```python
from build123d import *

# Parameters (mm, degrees)
SKETCH2_R           = 25
BOSS_EXTRUDE1_DEPTH = 12


with BuildPart() as part:
    # Sketch2 → Boss-Extrude1 (new body)
    with BuildSketch(Plane.XY):
        with BuildLine():
            Line((-2.137931034, 28.911787374), (1.862068966, 28.911787374))
            Line((1.862068966, 28.911787374), (1.862068966, 26.935714194))
            ThreePointArc((1.862068966, 26.935714194), (2.42026134, 26.891305938), (2.977412735, 26.835331438))
            Line((2.977412735, 26.835331438), (3.058825373, 28.828905384))
            Line((3.058825373, 28.828905384), (6.994543728, 28.114677805))
            Line((6.994543728, 28.114677805), (6.641702237, 26.170360934))
            ThreePointArc((6.641702237, 26.170360934), (7.18299483, 26.026997239), (7.72119794, 25.87243905))
            Line((7.72119794, 25.87243905), (8.157268617, 27.819438654))
            Line((8.157268617, 27.819438654), (11.9022081, 26.413939357))
            Line((11.9022081, 26.413939357), (11.207865734, 24.563870739))
            ThreePointArc((11.207865734, 24.563870739), (11.714860956, 24.326159433), (12.21681749, 24.077985182))
            Line((12.21681749, 24.077985182), (12.993530536, 25.915832275))
            Line((12.993530536, 25.915832275), (16.42732571, 23.864235166))
            Line((16.42732571, 23.864235166), (15.413799204, 22.167877528))
            ThreePointArc((15.413799204, 22.167877528), (15.870201812, 21.843458848), (16.319778474, 21.509645059))
            Line((16.319778474, 21.509645059), (17.412169691, 23.179269724))
            Line((17.412169691, 23.179269724), (20.424455555, 20.54751482))
            Line((20.424455555, 20.54751482), (19.124320485, 19.059390494))
            ThreePointArc((19.124320485, 19.059390494), (19.515461323, 18.658691523), (19.89820835, 18.249967246))
            Line((19.89820835, 18.249967246), (21.271167387, 19.697706372))
            Line((21.271167387, 19.697706372), (23.765126594, 16.570380442))
            Line((23.765126594, 16.570380442), (22.22017037, 15.338318966))
            ThreePointArc((22.22017037, 15.338318966), (22.53347785, 14.874218499), (22.837093437, 14.403720469))
            Line((22.837093437, 14.403720469), (24.44649226, 15.583042529))
            Line((24.44649226, 15.583042529), (26.34196691, 12.060660402))
            Line((26.34196691, 12.060660402), (24.601845697, 11.124261247))
            ThreePointArc((24.601845697, 11.124261247), (24.827249859, 10.611675855), (25.041975551, 10.094526265))
            Line((25.041975551, 10.094526265), (26.836086758, 10.967526878))
            Line((26.836086758, 10.967526878), (28.072154735, 7.163300813))
            Line((28.072154735, 7.163300813), (26.192797461, 6.552660618))
            ThreePointArc((26.192797461, 6.552660618), (26.323053629, 6.008065217), (26.441987966, 5.460885681))
            Line((26.441987966, 5.460885681), (28.363147346, 5.999505889))
            Line((28.363147346, 5.999505889), (28.900080409, 2.035706842))
            Line((28.900080409, 2.035706842), (26.941891163, 1.770452086))
            ThreePointArc((26.941891163, 1.770452086), (26.972812797, 1.211350419), (26.992133131, 0.651727738))
            Line((26.992133131, 0.651727738), (28.978593042, 0.838655845))
            Line((28.978593042, 0.838655845), (28.79913372, -3.157316422))
            Line((28.79913372, -3.157316422), (26.825050314, -3.068660234))
            ThreePointArc((26.825050314, -3.068660234), (26.755643568, -3.624298177), (26.674728928, -4.17837727))
            Line((26.674728928, -4.17837727), (28.662642913, -4.349149289))
            Line((28.662642913, -4.349149289), (27.772559177, -8.248860938))
            Line((27.772559177, -8.248860938), (25.846030277, -7.809143288))
            ThreePointArc((25.846030277, -7.809143288), (25.67852594, -8.343458848), (25.499976989, -8.874185796))
            Line((25.499976989, -8.874185796), (27.425451857, -9.397169186))
            Line((27.425451857, -9.397169186), (25.853351731, -13.075280276))
            Line((25.853351731, -13.075280276), (24.036297561, -12.298634052))
            ThreePointArc((24.036297561, -12.298634052), (23.77607936, -12.794453887), (23.505634809, -13.284770688))
            Line((23.505634809, -13.284770688), (25.306784213, -14.143156333))
            Line((25.306784213, -14.143156333), (23.103196288, -17.481449348))
            Line((23.103196288, -17.481449348), (21.454018464, -16.392836598))
            ThreePointArc((21.454018464, -16.392836598), (21.109450027, -16.83422465), (20.755802185, -17.268372119))
            Line((20.755802185, -17.268372119), (22.374735702, -18.434570799))
            Line((22.374735702, -18.434570799), (19.610485106, -21.325750254))
            Line((19.610485106, -21.325750254), (18.182189561, -19.960159888))
            ThreePointArc((18.182189561, -19.960159888), (17.7643456, -20.332929582), (17.338861001, -20.696953862))
            Line((17.338861001, -20.696953862), (18.723544776, -22.133482991))
            Line((18.723544776, -22.133482991), (15.487476798, -24.484624))
            Line((15.487476798, -24.484624), (14.325970126, -22.885947216))
            ThreePointArc((14.325970126, -22.885947216), (13.84828049, -23.178117427), (13.364634558, -23.460318479))
            Line((13.364634558, -23.460318479), (14.470563714, -25.121006829))
            Line((14.470563714, -25.121006829), (10.866688243, -26.856541785))
            Line((10.866688243, -26.856541785), (10.009302223, -25.076161369))
            ThreePointArc((10.009302223, -25.076161369), (9.48712025, -25.278341507), (8.960857764, -25.469649156))
            Line((8.960857764, -25.469649156), (9.752486829, -27.301120837))
            Line((9.752486829, -27.301120837), (5.896635386, -28.365268219))
            Line((5.896635386, -28.365268219), (5.370927111, -26.460407064))
            ThreePointArc((5.370927111, -26.460407064), (4.82103616, -26.566098892), (4.269071629, -26.660364353))
            Line((4.269071629, -26.660364353), (4.720956992, -28.603754358))
            Line((4.720956992, -28.603754358), (0.737059816, -28.962311594))
            Line((0.737059816, -28.962311594), (0.559925982, -26.994193503))
            ThreePointArc((0.559925982, -26.994193503), (0, -27), (-0.559925982, -26.994193503))
            Line((-0.559925982, -26.994193503), (-0.462308287, -28.987039679))
            Line((-0.462308287, -28.987039679), (-4.446205463, -28.628482443))
            Line((-4.446205463, -28.628482443), (-4.269071629, -26.660364353))
            ThreePointArc((-4.269071629, -26.660364353), (-4.82103616, -26.566098892), (-5.370927111, -26.460407064))
            Line((-5.370927111, -26.460407064), (-5.630714597, -28.438657694))
            Line((-5.630714597, -28.438657694), (-9.48656604, -27.374510312))
            Line((-9.48656604, -27.374510312), (-8.960857764, -25.469649156))
            ThreePointArc((-8.960857764, -25.469649156), (-9.48712025, -25.278341507), (-10.009302223, -25.076161369))
            Line((-10.009302223, -25.076161369), (-10.618145107, -26.976233851))
            Line((-10.618145107, -26.976233851), (-14.222020578, -25.240698895))
            Line((-14.222020578, -25.240698895), (-13.364634558, -23.460318479))
            ThreePointArc((-13.364634558, -23.460318479), (-13.84828049, -23.178117427), (-14.325970126, -22.885947216))
            Line((-14.325970126, -22.885947216), (-15.264299696, -24.646771656))
            Line((-15.264299696, -24.646771656), (-18.500367674, -22.295630647))
            Line((-18.500367674, -22.295630647), (-17.338861001, -20.696953862))
            ThreePointArc((-17.338861001, -20.696953862), (-17.7643456, -20.332929582), (-18.182189561, -19.960159888))
            Line((-18.182189561, -19.960159888), (-19.419847134, -21.525141941))
            Line((-19.419847134, -21.525141941), (-22.18409773, -18.633962486))
            Line((-22.18409773, -18.633962486), (-20.755802185, -17.268372119))
            ThreePointArc((-20.755802185, -17.268372119), (-21.109450027, -16.83422465), (-21.454018464, -16.392836598))
            Line((-21.454018464, -16.392836598), (-22.951224707, -17.711676453))
            Line((-22.951224707, -17.711676453), (-25.154812632, -14.373383438))
            Line((-25.154812632, -14.373383438), (-23.505634809, -13.284770688))
            ThreePointArc((-23.505634809, -13.284770688), (-23.77607936, -12.794453887), (-24.036297561, -12.298634052))
            Line((-24.036297561, -12.298634052), (-25.744931032, -13.32894311))
            Line((-25.744931032, -13.32894311), (-27.317031159, -9.65083202))
            Line((-27.317031159, -9.65083202), (-25.499976989, -8.874185796))
            ThreePointArc((-25.499976989, -8.874185796), (-25.67852594, -8.343458848), (-25.846030277, -7.809143288))
            Line((-25.846030277, -7.809143288), (-27.711174092, -8.517806569))
            Line((-27.711174092, -8.517806569), (-28.601257828, -4.61809492))
            Line((-28.601257828, -4.61809492), (-26.674728928, -4.17837727))
            ThreePointArc((-26.674728928, -4.17837727), (-26.755643568, -3.624298177), (-26.825050314, -3.068660234))
            Line((-26.825050314, -3.068660234), (-28.786757215, -3.432900716))
            Line((-28.786757215, -3.432900716), (-28.966216537, 0.56307155))
            Line((-28.966216537, 0.56307155), (-26.992133131, 0.651727738))
            ThreePointArc((-26.992133131, 0.651727738), (-26.972812797, 1.211350419), (-26.941891163, 1.770452086))
            Line((-26.941891163, 1.770452086), (-28.937110276, 1.762341391))
            Line((-28.937110276, 1.762341391), (-28.400177213, 5.726140438))
            Line((-28.400177213, 5.726140438), (-26.441987966, 5.460885681))
            ThreePointArc((-26.441987966, 5.460885681), (-26.323053629, 6.008065217), (-26.192797461, 6.552660618))
            Line((-26.192797461, 6.552660618), (-28.157400803, 6.900940395))
            Line((-28.157400803, 6.900940395), (-26.921332825, 10.70516646))
            Line((-26.921332825, 10.70516646), (-25.041975551, 10.094526265))
            ThreePointArc((-25.041975551, 10.094526265), (-24.827249859, 10.611675855), (-24.601845697, 11.124261247))
            Line((-24.601845697, 11.124261247), (-26.4726893, 11.817737496))
            Line((-26.4726893, 11.817737496), (-24.57721465, 15.340119624))
            Line((-24.57721465, 15.340119624), (-22.837093437, 14.403720469))
            ThreePointArc((-22.837093437, 14.403720469), (-22.53347785, 14.874218499), (-22.22017037, 15.338318966))
            Line((-22.22017037, 15.338318966), (-23.937123781, 16.354702791))
            Line((-23.937123781, 16.354702791), (-21.443164573, 19.482028721))
            Line((-21.443164573, 19.482028721), (-19.89820835, 18.249967246))
            ThreePointArc((-19.89820835, 18.249967246), (-19.515461323, 18.658691523), (-19.124320485, 19.059390494))
            Line((-19.124320485, 19.059390494), (-20.632199408, 20.366014482))
            Line((-20.632199408, 20.366014482), (-17.619913544, 22.997769386))
            Line((-17.619913544, 22.997769386), (-16.319778474, 21.509645059))
            ThreePointArc((-16.319778474, 21.509645059), (-15.870201812, 21.843458848), (-15.413799204, 22.167877528))
            Line((-15.413799204, 22.167877528), (-16.66413917, 23.72274571))
            Line((-16.66413917, 23.72274571), (-13.230343996, 25.774342819))
            Line((-13.230343996, 25.774342819), (-12.21681749, 24.077985182))
            ThreePointArc((-12.21681749, 24.077985182), (-11.714860956, 24.326159433), (-11.207865734, 24.563870739))
            Line((-11.207865734, 24.563870739), (-12.160479788, 26.317008371))
            Line((-12.160479788, 26.317008371), (-8.415540306, 27.722507668))
            Line((-8.415540306, 27.722507668), (-7.72119794, 25.87243905))
            ThreePointArc((-7.72119794, 25.87243905), (-7.18299483, 26.026997239), (-6.641702237, 26.170360934))
            Line((-6.641702237, 26.170360934), (-7.26597258, 28.06542073))
            Line((-7.26597258, 28.06542073), (-3.330254225, 28.779648309))
            Line((-3.330254225, 28.779648309), (-2.977412735, 26.835331438))
            ThreePointArc((-2.977412735, 26.835331438), (-2.42026134, 26.891305938), (-1.862068966, 26.935714194))
            Line((-1.862068966, 26.935714194), (-2.137931034, 28.911787374))
        make_face()
        Circle(SKETCH2_R, mode=Mode.SUBTRACT)
    extrude(amount=BOSS_EXTRUDE1_DEPTH)


solid = part.part
```
Verification items for the finished model (mm, model axes). A direction names the side the tool comes from. Coordinates: 2 decimals unless noted, no trailing zeros. Answer as a JSON object with one key per item and string values. Group by question number.
(1) Gauge pin test, flat ends, axial feed: pin 1 (8 mm diameter, centred on x = 18.5, y = -3, fed in from -Z); pin 2 (2 mm diameter, centred on y = 12, z = 4.5, fed in from +X); pin 3 (1 mm diameter, centred on y = -21, z = 7.5, fed in from +X). Record the tip position at first contact, or that the pin passes through.
(2) Tool access check on faces 1 (the face through (-27.993, 0.607, 5.916)), 2 (the face through (24.394, -13.708, 5.916)), 3 (the face through (12.69, -25.98, 5.92)), 4 (the face through (5.64, -27.43, 5.92)), 5 (the face through (-19.868, 19.704, 5.916)). Record the directions out of +Z, -Z, +X, -X, +Y, -Y that give a thin tool (end or side, any length) a straight path to the whole face; none if there is none.
(3) Release check for a two-part mould opening along Y. For faces 6 (the face through (-19.15, 21.66, 5.92)), 7 (the face through (22.29, -16.945, 5.916)), 8 (the face through (13, 22, 12)) record: +Y half, -Y half, draft (parallel to the pull), parting line (faces both ways), or undercut.
(4) Material ranges on line 1 (Y direction, x = 0, z = 8); line 2 (Y direction, x = 15.5, z = 7.25); line 3 (Y direction, x = 14, z = 2), recorded low to high.
Reply:
{
 "1": {"pin 1": "through", "pin 2": "x = 26.34", "pin 3": "x = 20.4"},
 "2": {"face 1": "+Z, -Z, -X", "face 2": "+Z, -Z, +X", "face 3": "+Z, -Z, +X, -Y", "face 4": "+Z, -Z, -Y", "face 5": "+Z, -Z"},
 "3": {"face 6": "+Y half", "face 7": "undercut", "face 8": "draft"},
 "4": {"line 1": "-27 to -25, 25 to 28.91", "line 2": "-24.48 to -19.62, 19.62 to 22.11, 22.31 to 24.42", "line 3": "-25.35 to -24.41, -23.09 to -20.71, 20.71 to 25.31"}
}
